For this review, take the finished solid that the model builds, in its own axes (mm). Give positions to 0.01 mm unless a question says otherwise; leave off trailing zeros. Write each loop counter-clockwise with the first axis right and the second up, starting at its lowest first coordinate (ties: lowest second). Pieces come first, ordered by that corner, then holes. Notation, with made-up numbers: M 17.25,74.25 L 37.25,74.25 A11 cw 37.25,89.25 Z; hole C 48,85 d11. An arc over 180 degrees is marked long. Answer as a JSON object with one key per item and string values. Group by question number.
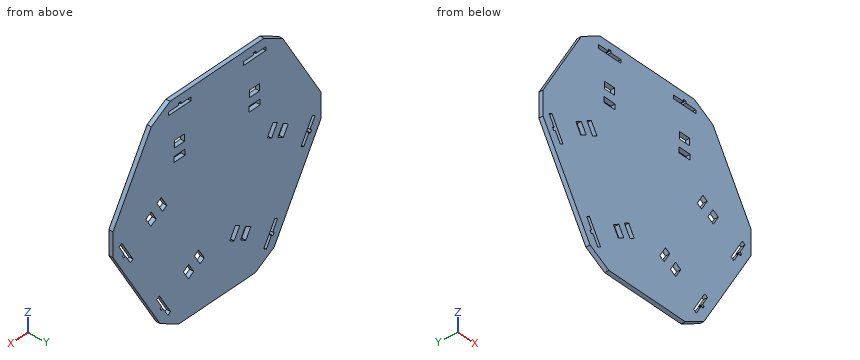
```python
from build123d import *

# Parameters (mm, degrees)
BOSS_EXTRUDE1_DEPTH           = 3
CUT_EXTRUDE1_DEPTH            = 119.131594354
SKETCH4_W                     = 8
SKETCH4_H                     = 5
SKETCH4_W_2                   = 9
SKETCH4_H_2                   = 4
CUT_EXTRUDE2_DEPTH            = 119.131594354
CIRPATTERN1_COUNT             = 3
CIRPATTERN1_COPY_1_DEPTH      = 119.131594354
CIRPATTERN1_COPY_2_DEPTH      = 119.131594354
CIRPATTERN1_COPY_3_SKETCH_W   = 8
CIRPATTERN1_COPY_3_SKETCH_H   = 5
CIRPATTERN1_COPY_3_SKETCH_W_2 = 9
CIRPATTERN1_COPY_3_SKETCH_H_2 = 4
CIRPATTERN1_COPY_3_DEPTH      = 119.131594354
CIRPATTERN1_COPY_4_SKETCH_W   = 8
CIRPATTERN1_COPY_4_SKETCH_H   = 5
CIRPATTERN1_COPY_4_SKETCH_W_2 = 9
CIRPATTERN1_COPY_4_SKETCH_H_2 = 4
CIRPATTERN1_COPY_4_DEPTH      = 119.131594354
CHAMFER1_SIZE                 = 10


with BuildPart() as part:
    # Sketch1 → Boss-Extrude1 (new body)
    with BuildSketch(Plane(origin=(0, 0, 0), x_dir=(1, 0, 0), z_dir=(0, 1, 0))):
        Polygon((-40.639997478, 78.456126624), (40.640002522, 78.456126624), (88.264992433, -4.032793087), (47.625005045, -74.423333537), (-47.625, -74.423333537), (-88.264997478, -4.032793087), align=None)
    extrude(amount=BOSS_EXTRUDE1_DEPTH)

    # Sketch2 → Cut-Extrude1 (cut, through all)
    with BuildSketch(Plane(origin=(0, 3, 0), x_dir=(1, 0, 0), z_dir=(0, 1, 0))):
        Polygon((29, -68), (29, -69.5), (31, -69.5), (31, -68), (38.96, -68), (38.96, -65.48), (21.04, -65.48), (21.04, -68), align=None)
    cut_extrude1 = extrude(amount=-CUT_EXTRUDE1_DEPTH, mode=Mode.SUBTRACT)

    # Sketch4 → Cut-Extrude2 (cut, through all)
    with BuildSketch(Plane(origin=(0, 3, 0), x_dir=(1, 0, 0), z_dir=(0, 1, 0))):
        with Locations((30, -43.68)):
            Rectangle(SKETCH4_W, SKETCH4_H)
        with Locations((30, -33.68)):
            Rectangle(SKETCH4_W_2, SKETCH4_H_2)
    cut_extrude2 = extrude(amount=-CUT_EXTRUDE2_DEPTH, mode=Mode.SUBTRACT)

    # Mirror1: Cut-Extrude1, Cut-Extrude2 across plane
    add(cut_extrude1.mirror(Plane(origin=(0, 0, 0), x_dir=(0, 0, 1), z_dir=(1, 0, 0))), mode=Mode.SUBTRACT)
    add(cut_extrude2.mirror(Plane(origin=(0, 0, 0), x_dir=(0, 0, 1), z_dir=(1, 0, 0))), mode=Mode.SUBTRACT)

    # CirPattern1: Cut-Extrude1, Cut-Extrude2 ×3 about axis
    cirpattern1_axis = Axis((0, 0, 0), (0, 1, 0))
    add([cut_extrude1.rotate(cirpattern1_axis, i * 360 / CIRPATTERN1_COUNT) for i in range(1, CIRPATTERN1_COUNT)], mode=Mode.SUBTRACT)
    add([cut_extrude2.rotate(cirpattern1_axis, i * 360 / CIRPATTERN1_COUNT) for i in range(1, CIRPATTERN1_COUNT)], mode=Mode.SUBTRACT)

    # CirPattern1 copy 1 sketch → CirPattern1 copy 1 (cut, through all)
    with BuildSketch(Plane(origin=(0, 3, 0), x_dir=(0.4999999999999998, 0, 0.8660254037844387), z_dir=(0, 1, 0))):
        Polygon((29, 68), (29, 69.5), (31, 69.5), (31, 68), (38.96, 68), (38.96, 65.48), (21.04, 65.48), (21.04, 68), align=None)
    extrude(amount=-CIRPATTERN1_COPY_1_DEPTH, mode=Mode.SUBTRACT)

    # CirPattern1 copy 2 sketch → CirPattern1 copy 2 (cut, through all)
    with BuildSketch(Plane(origin=(0, 3, 0), x_dir=(0.5000000000000004, 0, -0.8660254037844384), z_dir=(0, 1, 0))):
        Polygon((29, 68), (29, 69.5), (31, 69.5), (31, 68), (38.96, 68), (38.96, 65.48), (21.04, 65.48), (21.04, 68), align=None)
    extrude(amount=-CIRPATTERN1_COPY_2_DEPTH, mode=Mode.SUBTRACT)

    # CirPattern1 copy 3 sketch → CirPattern1 copy 3 (cut, through all)
    with BuildSketch(Plane(origin=(0, 3, 0), x_dir=(0.4999999999999998, 0, 0.8660254037844387), z_dir=(0, 1, 0))):
        with Locations((30, 43.68)):
            Rectangle(CIRPATTERN1_COPY_3_SKETCH_W, CIRPATTERN1_COPY_3_SKETCH_H)
        with Locations((30, 33.68)):
            Rectangle(CIRPATTERN1_COPY_3_SKETCH_W_2, CIRPATTERN1_COPY_3_SKETCH_H_2)
    extrude(amount=-CIRPATTERN1_COPY_3_DEPTH, mode=Mode.SUBTRACT)

    # CirPattern1 copy 4 sketch → CirPattern1 copy 4 (cut, through all)
    with BuildSketch(Plane(origin=(0, 3, 0), x_dir=(0.5000000000000004, 0, -0.8660254037844384), z_dir=(0, 1, 0))):
        with Locations((30, 43.68)):
            Rectangle(CIRPATTERN1_COPY_4_SKETCH_W, CIRPATTERN1_COPY_4_SKETCH_H)
        with Locations((30, 33.68)):
            Rectangle(CIRPATTERN1_COPY_4_SKETCH_W_2, CIRPATTERN1_COPY_4_SKETCH_H_2)
    extrude(amount=-CIRPATTERN1_COPY_4_DEPTH, mode=Mode.SUBTRACT)

    # Chamfer1
    chamfer1_edges = [part.edges().sort_by_distance(p)[0] for p in [
        (-40.639997478, 1.5, -78.456126624),
        (40.640002522, 1.5, -78.456126624),
        (88.264992433, 1.5, 4.032793087),
        (47.625005045, 1.5, 74.423333537),
        (-47.625, 1.5, 74.423333537),
        (-88.264997478, 1.5, 4.032793087),
    ]]
    chamfer(chamfer1_edges, length=CHAMFER1_SIZE)


solid = part.part
```
Item 1: Consider section C-C (z = 26). Give the boundary of the cut face in (x, y).
Item 2: Insertion check: P1, Ø0.9, axis at x = -31.5, y = 1.5, coming from the -Z side; P2, Ø1.6, axis at y = 2, z = 69, coming from the -X side; P3, Ø1.5, axis at x = 66.5, z = 20.5, coming from the -Y side. Each pin has a flat end and moves straight along its axis. Give the tip position at first contact, or say it passes through.
Item 3: To check wall thickness, follow probe 1 along Z at (x, y) = (28, 2.45); probe 2 along Z at (x, y) = (38.5, 0.3); probe 3 along X at (y, z) = (0.25, -39). State the ranges of each line that lie inside material, in increasing order.
Item 4: Consider section B-B (y = 1.8). State how many separate pieces and enclosed holes the cut face has, plus the area to 3 significant figures.
Item 5: Consider section A-A (x = 55). Give the boundary of the cut face in (y, z).
Result set:
{
 "1": {"outline": "M -75.58,0 L 75.58,0 L 75.58,3 L -75.58,3 Z"},
 "2": {"P1": "stops at z = -78.22", "P2": "stops at x = -48.4", "P3": "stops at y = 0"},
 "3": {"probe 1": "z = -78.46 to 31.68, 35.68 to 41.18, 46.18 to 65.48, 68 to 74.42", "probe 2": "z = -73.92 to -67.22, -64.28 to 65.48, 68 to 73.92", "probe 3": "x = -63.42 to -16.55, -14.06 to 14.06, 16.55 to 63.42"},
 "4": {"separate pieces": "1", "enclosed holes": "18", "area": "19,200 mm^2"},
 "5": {"outline": "M 0,-53.58 L 3,-53.58 L 3,2.9 L 0,2.9 Z; M 0,7.51 L 3,7.51 L 3,61.65 L 0,61.65 Z"}
}
